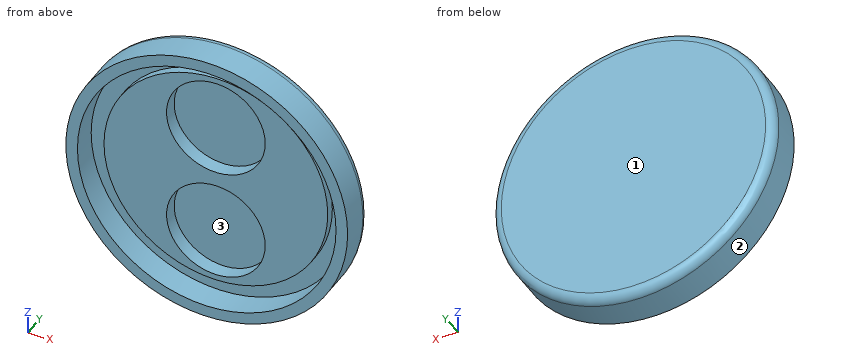
Autodesk Inventor part; units mm, degrees
ref_plane "YZ Plane" through (0, 0, 0) normal (1, 0, 0) x (0, 1, 0)
ref_plane "XZ Plane" through (0, 0, 0) normal (0, 1, 0) x (-1, 0, 0)
ref_plane "XY Plane" through (0, 0, 0) normal (0, 0, 1) x (1, 0, 0)
sketch "Sketch2" plane through (0, 0, 0) normal (0, 0, 1) x (1, 0, 0)
  line L0 (0, 0) -> (48.55, 0)
  line L1 (48.55, 0) -> (48.55, -13)
  line L2 (48.55, -13) -> (44.55, -13)
  line L3 (44.55, -13) -> (44.55, -4)
  line L4 (44.55, -4) -> (38.55, -4)
  line L5 (38.55, -4) -> (38.55, -7)
  line L6 (38.55, -7) -> (0, -7)
  line L7 (0, -7) -> (0, 0)
  dimension "d0" = 48.55
  dimension "d1" = 4
  dimension "d2" = 6
  dimension "d3" = 13
  dimension "d4" = 4
  dimension "d5" = 7
revolve "Revolution1" add sketch "Sketch2" angle 360 about axis through (0, -7, 0) along (0, 1, 0)
fillet "Fillet1" radius 3 1 edges at (-48.55, 0, 0)
sketch "Sketch3" plane through (0, -7, 0) normal (0, -1, 0) x (1, 0, 0)
  circle A0 centre (0, -19.55) radius 17
  circle A1 centre (0, 0) radius 38.55
  circle A2 centre (0, 19.55) radius 17
  dimension "d8" = 34
  dimension "d11" = 360
  dimension "d15" = 19.55
extrude "Extrusion1" cut sketch "Sketch3" against normal blind 5 contours A0 | A2
properties part number "lid-v1"
Work out the finished part from the listing and answer in its coordinate system (mm). Face numbers are marked on the shaded views. Give positions to 0.01 mm unless a question says otherwise; leave off trailing zeros. Loops run counter-clockwise (first coordinate to the right, second up) from the corner with the lowest first, then second, coordinate; pieces in that order, holes last. Notation, with made-up numbers: (9.5, 37.5) - (59.5, 37.5) arc R27 ccw to (59.5, 75.5) - close; hole circle Ø10 at (66.5, 67). An arc over 180 degrees is marked (long way). One line per question, with ' | ' between items.
(1) Straight lines are drawn through the part: probe 1 along X at (y, z) = (-6, 0); probe 2 along X at (y, z) = (-5, 29); probe 3 along X at (y, z) = (-9.25, 0). For each, find the intervals that lie inside material, in ascending order.
Recorded:
probe 1: x = -48.55 to -44.55, -38.55 to 38.55, 44.55 to 48.55 | probe 2: x = -38.94 to -33.82, -25.4 to -14.13, 14.13 to 25.4, 33.82 to 38.94 | probe 3: x = -48.55 to -44.55, 44.55 to 48.55
(2) The mould has two halves that part along X. Classify the marked faces 1, 2 and 3: +X half, -X half, draft (parallel to the pull), parting line (faces both ways), or undercut.
Recorded:
face 1: draft | face 2: parting line | face 3: undercut
(3) The part is cut by section A-A (z = 0). Write down the section's boundary in (x, y).
Recorded:
outline: (-48.55, -13) - (-44.55, -13) - (-44.55, -4) - (-38.55, -4) - (-38.55, -7) - (38.55, -7) - (38.55, -4) - (44.55, -4) - (44.55, -13) - (48.55, -13) - (48.55, -3) arc R3 ccw to (45.55, 0) - (-45.55, 0) arc R3 ccw to (-48.55, -3) - close
(4) The part is cut by section B-B (x = 0). Write down the section's boundary in (y, z).
Recorded:
outline: (-13, -48.55) - (-3, -48.55) arc R3 ccw to (0, -45.55) - (0, 45.55) arc R3 ccw to (-3, 48.55) - (-13, 48.55) - (-13, 44.55) - (-4, 44.55) - (-4, 38.55) - (-7, 38.55) - (-7, 36.55) - (-2, 36.55) - (-2, 2.55) - (-7, 2.55) - (-7, -2.55) - (-2, -2.55) - (-2, -36.55) - (-7, -36.55) - (-7, -38.55) - (-4, -38.55) - (-4, -44.55) - (-13, -44.55) - close
(5) Each of these flat-tipped pins is pushed along its axis until it touches: pin 1 Ø10 at (x, z) = (37.5, -11) entering from +Y; pin 2 Ø3 at (y, z) = (-4.5, -26.5) entering from -X; pin 3 Ø23 at (x, z) = (-15.5, 15.5) entering from -Y; pin 4 Ø17 at (x, z) = (7.5, -19.5) entering from -Y. Where does it stop, or does it pass through?
Recorded:
pin 1: stops at y = 0 | pin 2: stops at x = -41.62 | pin 3: stops at y = -7 | pin 4: stops at y = -2
(6) The part is cut by section C-C (y = -10.5). Write down the section's boundary in (x, z).
Recorded:
outline: circle Ø97.1 at (0, 0); hole circle Ø89.1 at (0, 0)
